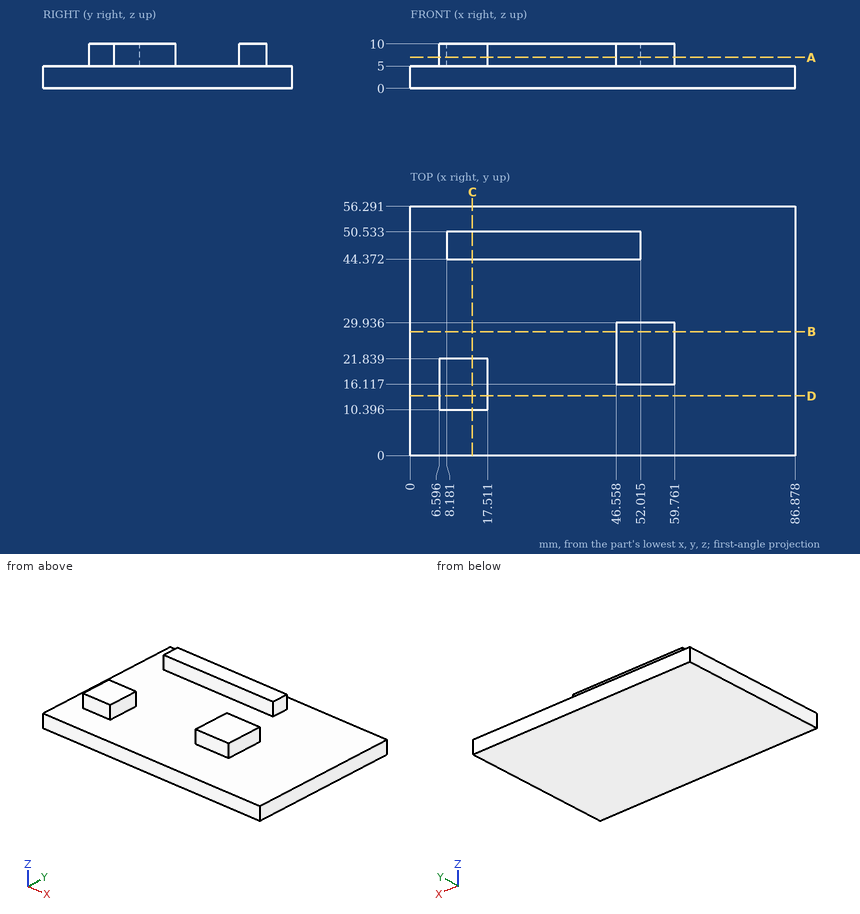
Print and shaded views of the part. All mm, measured from the part's lowest x, y and z. Coordinates: 2 decimals unless noted, no trailing zeros. Write each loop counter-clockwise with the first axis right and the second up, starting at its lowest first coordinate (ties: lowest second). Pieces come first, ordered by that corner, then holes.
(1) Cut at D-D, the plane y = 13.5. List the corners of the cut face in (x, z), and give its area (3 significant figures).
(2) Flat gauge pins, fed straight in: pin 1 (1.5 mm diameter, centred on y = 14, z = 8, fed in from +X); pin 2 (1.5 mm diameter, centred on y = 24.5, z = 7, fed in from -X); pin 3 (2.5 mm diameter, centred on x = 54, z = 7, fed in from +Y); pin 4 (17 mm diameter, centred on x = 43, y = 35, fed in from +Z). Where does each tip first touch, or does it go through?
(3) Cut at C-C, the plane x = 14. List the corners of the cut face in (y, z) (1 decimal).
(4) Drill centre lines: probe 1 along Z at (x, y) = (53, 50.5); probe 2 along X at (y, z) = (29.5, 9.25); probe 3 along Y at (x, z) = (27.5, 9.25). Where is each one in solid material? Low to high.
(5) Cut at A-A, the plane z = 7. List the corners of the cut face in (x, y) (1 decimal).
(6) Cut at B-B, the plane y = 28. List the corners of the cut face in (x, z).
Geometry says:
1. outline: (0, 0) - (86.88, 0) - (86.88, 5) - (17.51, 5) - (17.51, 10) - (6.6, 10) - (6.6, 5) - (0, 5) - close
1. area: 489 mm2
2. pin 1: stops at x = 17.51
2. pin 2: stops at x = 46.56
2. pin 3: stops at y = 29.94
2. pin 4: stops at z = 10
3. outline: (0, 0) - (56.3, 0) - (56.3, 5) - (50.5, 5) - (50.5, 10) - (44.4, 10) - (44.4, 5) - (21.8, 5) - (21.8, 10) - (10.4, 10) - (10.4, 5) - (0, 5) - close
4. probe 1: z = 0 to 5
4. probe 2: x = 46.56 to 59.76
4. probe 3: y = 44.37 to 50.53
5. outline: (6.6, 10.4) - (17.5, 10.4) - (17.5, 21.8) - (6.6, 21.8) - close; (8.2, 44.4) - (52, 44.4) - (52, 50.5) - (8.2, 50.5) - close; (46.6, 16.1) - (59.8, 16.1) - (59.8, 29.9) - (46.6, 29.9) - close
6. outline: (0, 0) - (86.88, 0) - (86.88, 5) - (59.76, 5) - (59.76, 10) - (46.56, 10) - (46.56, 5) - (0, 5) - close
